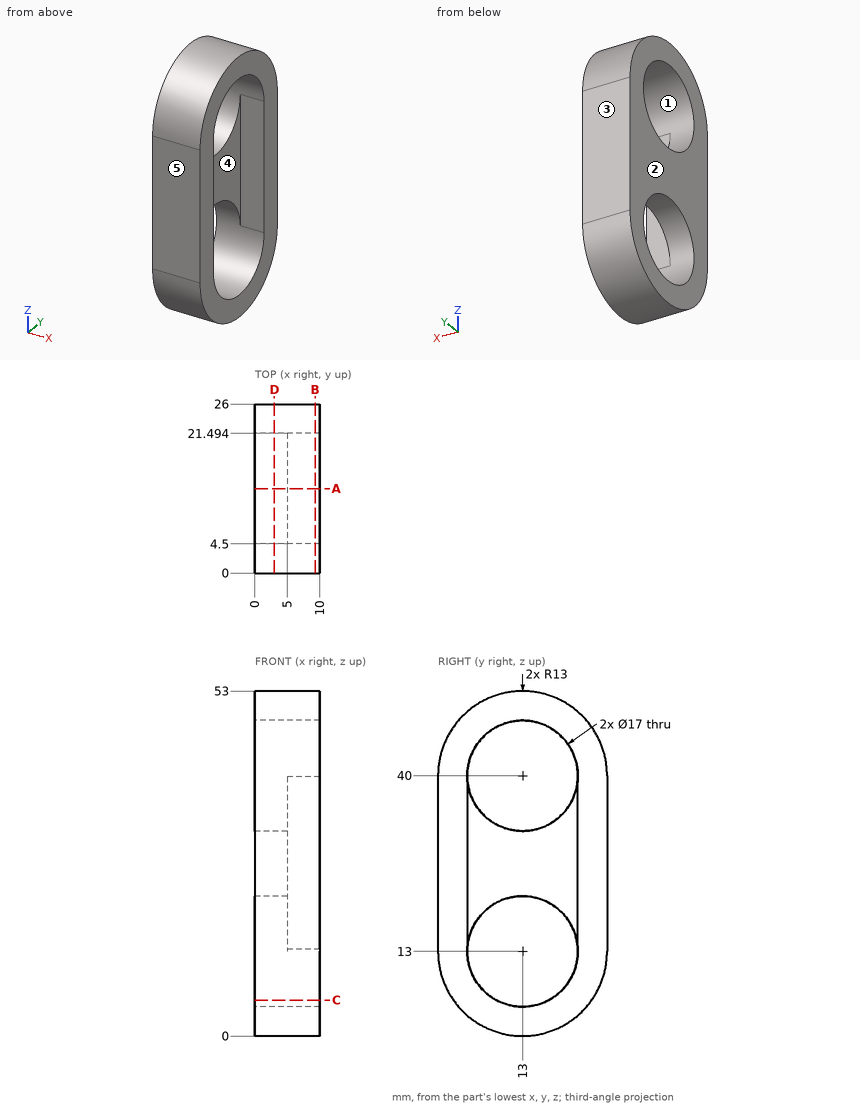
Geometry: see drawing. Coordinates: mm, zero at the bounding-box minimum. A direction names the side the tool comes from. Give positions to 0.01 mm unless a question says otherwise; leave off trailing zeros. Write each loop counter-clockwise with the first axis right and the second up, starting at its lowest first coordinate (ties: lowest second). Pieces come first, ordered by that corner, then holes. Notation, with made-up numbers: M 44,60.25 L 75,60.25 A16 cw 75,88.25 Z; hole C -13,75.5 d4. An arc over 180 degrees is marked long. Return JSON: item names as keys, results as strings. Group by question number.
1) Cut plane D-D, the plane x = 3. Output: boundary loops of the cut face in (y, z), then the cut area to 3 significant figures.
2) First-contact query: pin 1 Ø13.5 at (y, z) = (13.5, 20.5) entering from +X; pin 2 Ø3 at (x, y) = (6, 22.5) entering from +Z; pin 3 Ø4 at (x, y) = (2.5, 10.5) entering from +Z. Flat tips, straight axial feed; report the tip coordinate or a pass-through.
3) Cut plane B-B, the plane x = 9.25. Output: boundary loops of the cut face in (y, z).
4) Cut plane A-A, the plane y = 13. Output: boundary loops of the cut face in (x, z), then the cut area to 3 significant figures.
5) Ray query, L1, parallel to Z at x = 3.25, y = 13; L2, parallel to Y at x = 3.25, z = 40; L3, parallel to Z at x = 6.25, y = 13. Return the intervals inside material, ascending.
6) Cut plane C-C, the plane z = 5.5. Output: boundary loops of the cut face in (x, y).
7) Draft query along Y for the marked faces 1, 2 and 3. Return one class per face: released by +Y, released by -Y, zero draft, split by the parting line, or undercut.
8) Set-up query: the marked faces 4 and 5. Return all of +Z, -Z, +X, -X, +Y, -Y with unobstructed straight access to the full face (end or side cutting, diameter ignored); none if empty.
Data:
{
 "1": {"outline": "M 0,13 A13 ccw 26,13 L 26,40 A13 ccw 0,40 Z; hole C 13,13 d17; hole C 13,40 d17", "area": "779 mm²"},
 "2": {"pin 1": "stops at x = 5", "pin 2": "stops at z = 50.25", "pin 3": "stops at z = 52.99"},
 "3": {"outline": "M 0,13 A13 ccw 26,13 L 26,40 A13 ccw 0,40 Z; hole M 4.5,13 A8.5 ccw long 21.49,13.32 L 21.5,40 A8.5 ccw long 4.5,39.88 Z"},
 "4": {"outline": "M 0,0 L 10,0 L 10,4.5 L 0,4.5 Z; M 0,21.5 L 5,21.5 L 5,31.5 L 0,31.5 Z; M 0,48.5 L 10,48.5 L 10,53 L 0,53 Z", "area": "140 mm²"},
 "5": {"L1": "z = 0 to 4.5, 21.5 to 31.5, 48.5 to 53", "L2": "y = 0 to 4.5, 21.5 to 26", "L3": "z = 0 to 4.5, 48.5 to 53"},
 "6": {"outline": "M 0,2.38 L 10,2.38 L 10,9 L 0,9 Z; M 0,17 L 10,17 L 10,23.62 L 0,23.62 Z"},
 "7": {"face 1": "undercut", "face 2": "zero draft", "face 3": "released by +Y"},
 "8": {"face 4": "+X", "face 5": "+Z, -Z, +X, -X, -Y"}
}
